from build123d import *

# Parameters (mm, degrees)
SKETCH1_R           = 1
BOSS_EXTRUDE1_DEPTH = 4.2
SKETCH2_R           = 1.2
BOSS_EXTRUDE2_DEPTH = 4
SKETCH3_W           = 25
SKETCH3_H           = 4.2
BOSS_EXTRUDE3_DEPTH = 2
SKETCH4_W           = 25
SKETCH4_H           = 2
BOSS_EXTRUDE4_DEPTH = 0.6
BOSS_EXTRUDE5_START = -5.4
SKETCH1_3_R         = 1
BOSS_EXTRUDE5_DEPTH = 5.4
SKETCH4_2_W         = 25
SKETCH4_2_H         = 2
BOSS_EXTRUDE6_DEPTH = 5.4
CUT_EXTRUDE2_REACH  = 35.413
SKETCH5_W           = 25
SKETCH5_H           = 1.2
SKETCH6_W           = 2.096367106
SKETCH6_H           = 4.2
BOSS_EXTRUDE8_DEPTH = 21.5
SKETCH5_2_W         = 25
SKETCH5_2_H         = 1.2
CUT_EXTRUDE4_DEPTH  = 2.5
SKETCH8_R           = 1.2
SKETCH8_R_2         = 1.1
CUT_EXTRUDE5_DEPTH  = 3.2
CHAMFER1_SIZE       = 0.5
SKETCH10_W          = 0.4
SKETCH10_H          = 3.208969491
CUT_EXTRUDE6_DEPTH  = 2


# Read off the part's stored shape, not the designer's step: Mirror1
with BuildPart() as part:
    # Sketch1 → Boss-Extrude1 (new body)
    with BuildSketch(Plane(origin=(0, 0, 0), x_dir=(1, 0, 0), z_dir=(0, 1, 0))):
        Polygon((0, 0), (25, 0), (25, 24), (20.75, 24), (20.75, 2.5), (4.25, 2.5), (4.25, 24), (0, 24), align=None)
        with Locations(Location((2, 14.5, 0), (0, 0, 270))):
            Circle(SKETCH1_R, mode=Mode.SUBTRACT)
        with Locations(Location((2, 2, 0), (0, 0, 270))):
            Circle(SKETCH1_R, mode=Mode.SUBTRACT)
        with Locations(Location((23, 2, 0), (0, 0, 90))):
            Circle(SKETCH1_R, mode=Mode.SUBTRACT)
        with Locations(Location((23, 14.5, 0), (0, 0, 90))):
            Circle(SKETCH1_R, mode=Mode.SUBTRACT)
    extrude(amount=BOSS_EXTRUDE1_DEPTH)

    # Sketch2 → Boss-Extrude2 (add)
    with BuildSketch(Plane.ZY):
        with Locations((-14, 2.2)):
            Circle(SKETCH2_R)
    extrude(amount=BOSS_EXTRUDE2_DEPTH)

    # Sketch3 → Boss-Extrude3 (add)
    with BuildSketch(Plane.XY):
        with Locations((12.5, 2.1)):
            Rectangle(SKETCH3_W, SKETCH3_H)
    extrude(amount=BOSS_EXTRUDE3_DEPTH)

    # Sketch4 → Boss-Extrude4 (add)
    with BuildSketch(Plane.XZ):
        with Locations((12.5, 1)):
            Rectangle(SKETCH4_W, SKETCH4_H)
    extrude(amount=BOSS_EXTRUDE4_DEPTH)

    # Sketch1<3> → Boss-Extrude5 (add)
    with BuildSketch(Plane(origin=(0, 0, 0), x_dir=(1, 0, 0), z_dir=(0, 1, 0)).offset(BOSS_EXTRUDE5_START)):
        Polygon((0, 0), (25, 0), (25, 24), (20.75, 24), (20.75, 2.5), (4.25, 2.5), (4.25, 24), (0, 24), align=None)
        with Locations(Location((2, 14.5, 0), (0, 0, 270))):
            Circle(SKETCH1_3_R, mode=Mode.SUBTRACT)
        with Locations(Location((2, 2, 0), (0, 0, 270))):
            Circle(SKETCH1_3_R, mode=Mode.SUBTRACT)
        with Locations(Location((23, 2, 0), (0, 0, 90))):
            Circle(SKETCH1_3_R, mode=Mode.SUBTRACT)
        with Locations(Location((23, 14.5, 0), (0, 0, 90))):
            Circle(SKETCH1_3_R, mode=Mode.SUBTRACT)
    extrude(amount=BOSS_EXTRUDE5_DEPTH)

    # Sketch4<2> → Boss-Extrude6 (add)
    with BuildSketch(Plane.XZ):
        with Locations((12.5, 1)):
            Rectangle(SKETCH4_2_W, SKETCH4_2_H)
    extrude(amount=BOSS_EXTRUDE6_DEPTH)

    # Cut-Extrude2: up to this face of the body (flat: up to its plane)
    cut_extrude2_end = Plane(part.part.faces().sort_by_distance((22.875, -0.6, -24))[0])
    # Sketch5 → Cut-Extrude2 (cut, up to the picked face)
    with BuildSketch(Plane(origin=(0, 0, -2.5), x_dir=(-1, 0, 0), z_dir=(0, 0, -1)), mode=Mode.PRIVATE) as cut_extrude2_sk1:
        with Locations((-12.5, -0.6)):
            Rectangle(SKETCH5_W, SKETCH5_H)
    cut_extrude2_tool1 = split(extrude(cut_extrude2_sk1.sketch, amount=CUT_EXTRUDE2_REACH, mode=Mode.PRIVATE), bisect_by=cut_extrude2_end, keep=Keep.BOTH, mode=Mode.PRIVATE)
    add(cut_extrude2_tool1.solids().sort_by(Axis((12.5, -0.6, -2.5), (0, 0, -1)))[0], mode=Mode.SUBTRACT)

    # Sketch6 → Boss-Extrude8 (add)
    with BuildSketch(Plane(origin=(0, 0, -2.5), x_dir=(-1, 0, 0), z_dir=(0, 0, -1))):
        with Locations((-19.701816447, 2.1)):
            Rectangle(SKETCH6_W, SKETCH6_H)
        with Locations((-5.298183553, 2.1)):
            Rectangle(SKETCH6_W, SKETCH6_H)
        with Locations((-5.298183553, -3.3)):
            Rectangle(SKETCH6_W, SKETCH6_H)
        with Locations((-19.701816447, -3.3)):
            Rectangle(SKETCH6_W, SKETCH6_H)
    extrude(amount=BOSS_EXTRUDE8_DEPTH)

    # Sketch5<2> → Cut-Extrude4 (cut)
    with BuildSketch(Plane(origin=(0, 0, -2.5), x_dir=(-1, 0, 0), z_dir=(0, 0, -1))):
        with Locations((-12.5, -0.6)):
            Rectangle(SKETCH5_2_W, SKETCH5_2_H)
    extrude(amount=-CUT_EXTRUDE4_DEPTH, mode=Mode.SUBTRACT)

    # Sketch8 → Cut-Extrude5 (cut)
    with BuildSketch(Plane.ZY):
        with Locations((-14, 2.2)):
            Circle(SKETCH8_R)
        with Locations((-14, 2.2)):
            Circle(SKETCH8_R_2, mode=Mode.SUBTRACT)
    extrude(amount=CUT_EXTRUDE5_DEPTH, mode=Mode.SUBTRACT)

    # Chamfer1
    chamfer1_edges = [part.edges().sort_by_distance(p)[0] for p in [
        (-4, 2.2, -15.2),
    ]]
    chamfer(chamfer1_edges, length=CHAMFER1_SIZE)

    # Sketch10 → Cut-Extrude6 (cut)
    with BuildSketch(Plane.ZY.offset(4)):
        with Locations((-14, 2.169354983)):
            Rectangle(SKETCH10_W, SKETCH10_H)
    extrude(amount=-CUT_EXTRUDE6_DEPTH, mode=Mode.SUBTRACT)

    # Mirror1: part across plane


with BuildPart() as part_1:
    add(part.part)
    add(part.part.mirror(Plane.ZY.offset(-12.5)))


solid = part_1.part
Check sheet for the modelled part. Datum: model origin and axes. Units: mm. A direction names the side the tool comes from. Give positions to 0.01 mm unless a question says otherwise; leave off trailing zeros. Loops run counter-clockwise (first coordinate to the right, second up) from the corner with the lowest first, then second, coordinate; pieces in that order, holes last. Notation, with made-up numbers: M 43.5,26 L 97.5,26 A34 cw 97.5,62 Z; hole C 40.5,81 d2. An arc over 180 degrees is marked long. Use a Markdown table: item, result. Add a question column.
Q1. Tool access check on faces 3 (the flat face through (13, -3, -2.5)), 4 (the flat face through (21, 0, -12)), 5 (the cylindrical face through (-3.35, 2.22, -15.2)), 6 (the flat face through (28, 2, -14.2)), 7 (the cylindrical face through (28.35, 2.22, -15.2)). Record the directions out of +Z, -Z, +X, -X, +Y, -Y that give a thin tool (end or side, any length) a straight path to the whole face; none if there is none.
Q2. Sectioned sample at D-D, the plane z = -7.75. Record the cut outline in (x, y), then the cut area to 3 significant figures.
Q3. Sectioned sample at A-A, the plane z = -2. Record the cut outline in (x, y).
Q4. Sectioned sample at B-B, the plane x = 23. Record the cut outline in (y, z), then the cut area to 3 significant figures.
Q5. Sectioned sample at C-C, the plane y = -3. Record the cut outline in (x, z), then the cut area to 3 significant figures.
Q6. Go/stop test with flat-tipped pins: pin 1 (3 mm diameter, centred on x = 8, y = 2, fed in from -Z); pin 2 (1.3 mm diameter, centred on y = -3.5, z = -10.5, fed in from +X); pin 3 (5 mm diameter, centred on y = 1, z = -19, fed in from -X). Record where each tip stops, or that it passes through.
Q7. Scan lines: line 1 along Z through (x, y) = (2, -4.2); line 2 along X through (y, z) = (1.7, -2); line 3 along X through (y, z) = (-3.35, -14.5). Record each from-to range of solid material in increasing order. Write a range as [from, to].
Q8. Mould release check, pull along X, two halves, no side actions. Record for faces 1 (the flat face through (21, -5.4, -11)), 2 (the cylindrical face through (24, 2, -2)): pulls with the +X half, pulls with the -X half, needs draft (parallel to the pull), parting line crosses it, or undercut.
Verdict:
| question | item | result |
|---|---|---|
| 1 | face 3 | -Z, +Y, -Y |
| 1 | face 4 | -Z, +X, -X |
| 1 | face 5 | -Z, -X |
| 1 | face 6 | +X, +Y, -Y |
| 1 | face 7 | -Z, +X |
| 2 | outline | M 0,-5.4 L 6.35,-5.4 L 6.35,-1.2 L 0,-1.2 Z; M 0,0 L 6.35,0 L 6.35,4.2 L 0,4.2 Z; M 18.65,-5.4 L 25,-5.4 L 25,-1.2 L 18.65,-1.2 Z; M 18.65,0 L 25,0 L 25,4.2 L 18.65,4.2 Z |
| 2 | area | 107 mm^2 |
| 3 | outline | M 0,-5.4 L 1,-5.4 L 1,-1.2 L 0,-1.2 Z; M 0,0 L 1,0 L 1,4.2 L 0,4.2 Z; M 3,-5.4 L 22,-5.4 L 22,-1.2 L 3,-1.2 Z; M 3,0 L 22,0 L 22,4.2 L 3,4.2 Z; M 24,-5.4 L 25,-5.4 L 25,-1.2 L 24,-1.2 Z; M 24,0 L 25,0 L 25,4.2 L 24,4.2 Z |
| 4 | outline | M -5.4,-24 L -1.2,-24 L -1.2,-15.5 L -5.4,-15.5 Z; M -5.4,-13.5 L -1.2,-13.5 L -1.2,-3 L -5.4,-3 Z; M -5.4,-1 L -1.2,-1 L -1.2,0 L 0,0 L 0,-1 L 4.2,-1 L 4.2,2 L -5.4,2 Z; M 0,-24 L 4.2,-24 L 4.2,-15.5 L 0,-15.5 Z; M 0,-13.5 L 4.2,-13.5 L 4.2,-3 L 0,-3 Z |
| 4 | area | 187 mm^2 |
| 5 | outline | M 0,-24 L 6.35,-24 L 6.35,-2.5 L 18.65,-2.5 L 18.65,-24 L 25,-24 L 25,2 L 0,2 Z; hole C 2,-14.5 d2; hole C 2,-2 d2; hole C 23,-14.5 d2; hole C 23,-2 d2 |
| 5 | area | 373 mm^2 |
| 6 | pin 1 | z = -2.5 |
| 6 | pin 2 | x = 25 |
| 6 | pin 3 | x = 0 |
| 7 | line 1 | [-24, -15.5], [-13.5, -3], [-1, 2] |
| 7 | line 2 | [0, 1], [3, 22], [24, 25] |
| 7 | line 3 | [0, 1], [3, 6.35], [18.65, 22], [24, 25] |
| 8 | face 1 | needs draft |
| 8 | face 2 | undercut |
